Autodesk Fusion 360 part; units mm, degrees
sketch "Sketch2" plane through (0, 0, 0) normal (0, 1, 0) x (1, 0, 0)
  circle A0 centre (0, 0) radius 75
  dimension "d1" = 150
extrude "Extrude1" add sketch "Sketch2" along normal blind 200
fillet "Fillet1" radius 40 1 edges at (-69.9246, 0, 27.1212)
hole "Hole1" at (0, 200, 0) direction (0, -1, 0) diameter 120 depth 165 tip angle 118
hole "Hole2" at (75, 117.8728, 0) direction (-1, 0, 0) diameter 45.97 depth 50 tip angle 118
The model under review builds one solid part; all positions refer to its coordinate system, in mm. A direction names the side the tool comes from. Round coordinates to 2 decimals unless told otherwise and drop trailing zeros. Order: outer loops, then holes, each group sorted by start corner. A loop starts at its lowest first (then second) coordinate and runs counter-clockwise, first axis right, second up. Notation, with made-up numbers: (20.5, 61.25) - (47.5, 61.25) arc R26 cw to (47.5, 92.25) - close; hole circle Ø7 at (32.5, -24.75). An arc over 180 degrees is marked (long way). Use one line per item in the form item = value.
Q1. To check wall thickness, follow line 1 (Z direction, x = 0, y = 96.5); line 2 (Z direction, x = -16, y = 20); line 3 (X direction, y = 163, z = -39). State the ranges of each line that lie inside material, in increasing order.
Response values:
line_1 = -75 to -60, 60 to 75
line_2 = -67.78 to -31.17, 31.17 to 67.78
line_3 = -64.06 to -45.6, 45.6 to 64.06
Q2. Clearance check with flat-ended pins moving along their axes: P1, Ø12, axis at x = 13, z = 21.5, coming from the -Y side; P2, Ø12, axis at x = -14.5, z = 27, coming from the +Y side; P3, Ø10, axis at x = 23.5, y = 154, coming from the -Z side; P4, Ø10, axis at x = 2, z = -5, coming from the +Y side. State where each tip first meets the part, or that it passes through.
Response values:
P1 = 0
P2 = 20.97
P3 = -72.68
P4 = 5.19
Q3. Add section A-A on y = 48. Give the boundary of the cut face in (x, z), then the cut area to 3 significant figures.
Response values:
outline = circle Ø150 at (0, 0); hole circle Ø120 at (0, 0)
area = 6,360 mm^2
Q4. Mouldability with a two-part tool opening along X and no side actions: class faces 3 (the conical face through (1.62, 2.189, 5.145)), 4 (the cylindrical face through (-59.517, 118.88, -45.636)), 5 (the flat face through (-34, 200, -50)), 6 (the cylindrical face through (-59.49, 116.34, -7.81)) as pulls with the +X half, pulls with the -X half, needs draft (parallel to the pull), parting line crosses it, or undercut.
Response values:
face_3 = undercut
face_4 = parting line crosses it
face_5 = needs draft
face_6 = undercut
Q5. Tool access review of faces 1 (the flat face through (0, 0, 7)), 2 (the cylindrical face through (65.07, 126.68, -21.23)): name each direction out of +Z, -Z, +X, -X, +Y, -Y from which nothing blocks a thin tool from reaching the whole face with its end or side.
Response values:
face_1 = +Z, -Z, +X, -X, -Y
face_2 = +X
